```python
from build123d import *

# Parameters (mm, degrees)
BOSS_EXTRUDE1_DEPTH     = 15.21999998
SKETCH2_W               = 36.809677156
SKETCH2_H               = 26.071604974
BOSS_EXTRUDE2_DEPTH     = 3
SKETCH3_W               = 36.809677156
SKETCH3_H               = 26.071604974
BOSS_EXTRUDE3_DEPTH     = 2
SKETCH4_W               = 60.36112228
SKETCH4_H               = 157.574347664
SKETCH4_W_2             = 21
SKETCH4_H_2             = 111.767475737
CUT_EXTRUDE1_DEPTH      = 38.576
SKETCH5_W               = 10
SKETCH5_H               = 2
CUT_EXTRUDE2_DEPTH      = 38.576
SKETCH6_W               = 35.571492448
SKETCH6_H               = 20.32
CUT_EXTRUDE3_DEPTH      = 25.876
CUT_EXTRUDE3_DEPTH_BACK = 20.32
SKETCH7_W               = 25.588268566
SKETCH7_H               = 5
CUT_EXTRUDE4_DEPTH      = 25.876
SKETCH10_R              = 48.677475689
SKETCH10_R_2            = 20.5
CUT_EXTRUDE5_DEPTH      = 14.478
CUT_EXTRUDE5_DEPTH_BACK = 169.64
BOSS_EXTRUDE4_DEPTH     = 15.208
SKETCH12_W              = 30.501346117
SKETCH12_H              = 25.675497492
CUT_EXTRUDE8_DEPTH      = 8.604
CUT_EXTRUDE8_DEPTH_BACK = 0.0254
SKETCH13_W              = 21
SKETCH13_H              = 10.21999998
CUT_EXTRUDE9_DEPTH      = 8.604


with BuildPart() as part:
    # Sketch1 → Boss-Extrude1 (new body)
    with BuildSketch(Plane(origin=(0, 0, 0), x_dir=(1, 0, 0), z_dir=(0, 1, 0))):
        with BuildLine():
            Line((18.404838578, -7.300000132), (-18.404838578, -7.300000132))
            Line((-18.404838578, -7.300000132), (-18.404838578, 7.300000132))
            Line((-18.404838578, 7.300000132), (-18.404838578, 11.471604964))
            ThreePointArc((-18.404838578, 11.471604964), (0, 0), (18.404838578, 11.471604964))
            Line((18.404838578, 11.471604964), (18.404838578, 7.300000132))
            Line((18.404838578, 7.300000132), (18.404838578, -7.300000132))
        make_face()
    extrude(amount=BOSS_EXTRUDE1_DEPTH)

    # Sketch2 → Boss-Extrude2 (add)
    with BuildSketch(Plane(origin=(0, 15.21999998, 0), x_dir=(1, 0, 0), z_dir=(0, 1, 0))):
        with Locations((0, 5.735802355)):
            Rectangle(SKETCH2_W, SKETCH2_H)
    extrude(amount=-BOSS_EXTRUDE2_DEPTH)

    # Sketch3 → Boss-Extrude3 (add)
    with BuildSketch(Plane.XZ):
        with Locations((0, -5.735802355)):
            Rectangle(SKETCH3_W, SKETCH3_H)
    extrude(amount=-BOSS_EXTRUDE3_DEPTH)

    # Sketch4 → Cut-Extrude1 (cut)
    with BuildSketch(Plane.XZ):
        with Locations((0, -3.625194089)):
            Rectangle(SKETCH4_W, SKETCH4_H)
        with Locations((0, -3.62519409)):
            Rectangle(SKETCH4_W_2, SKETCH4_H_2, mode=Mode.SUBTRACT)
    extrude(amount=-CUT_EXTRUDE1_DEPTH, mode=Mode.SUBTRACT)

    # Sketch5 → Cut-Extrude2 (cut)
    with BuildSketch(Plane.XZ.offset(-12.21999998)):
        with Locations((0, -3.2352)):
            Rectangle(SKETCH5_W, SKETCH5_H)
    extrude(amount=-CUT_EXTRUDE2_DEPTH, mode=Mode.SUBTRACT)

    # Sketch6 → Cut-Extrude3 (cut, two sides)
    with BuildSketch(Plane.XZ.offset(-12.21999998)) as cut_extrude3_sk:
        with Locations((0, -18.771604842)):
            Rectangle(SKETCH6_W, SKETCH6_H)
    extrude(amount=CUT_EXTRUDE3_DEPTH, mode=Mode.SUBTRACT)
    extrude(cut_extrude3_sk.sketch, amount=-CUT_EXTRUDE3_DEPTH_BACK, mode=Mode.SUBTRACT)

    # Sketch7 → Cut-Extrude4 (cut)
    with BuildSketch(Plane(origin=(0, 15.21999998, 0), x_dir=(1, 0, 0), z_dir=(0, 1, 0))):
        with Locations((0, -7.300000132)):
            Rectangle(SKETCH7_W, SKETCH7_H)
    extrude(amount=-CUT_EXTRUDE4_DEPTH, mode=Mode.SUBTRACT)

    # Sketch10 → Cut-Extrude5 (cut, two sides)
    with BuildSketch(Plane(origin=(0, 15.21999998, 0), x_dir=(1, 0, 0), z_dir=(0, 1, 0))) as cut_extrude5_sk:
        with Locations((0, 18.199999842)):
            Circle(SKETCH10_R)
        with Locations((0, 18.199999842)):
            Circle(SKETCH10_R_2, mode=Mode.SUBTRACT)
    extrude(amount=CUT_EXTRUDE5_DEPTH, mode=Mode.SUBTRACT)
    extrude(cut_extrude5_sk.sketch, amount=-CUT_EXTRUDE5_DEPTH_BACK, mode=Mode.SUBTRACT)

    # Sketch11 → Boss-Extrude4 (add)
    with BuildSketch(Plane(origin=(0, 15.21999998, 0), x_dir=(1, 0, 0), z_dir=(0, 1, 0))):
        with BuildLine():
            Line((-10.5, 8.611604842), (10.5, 8.611604842))
            ThreePointArc((10.5, 8.611604842), (0, 11.50478798), (-10.5, 8.611604842))
        make_face()
    extrude(amount=-BOSS_EXTRUDE4_DEPTH)

    # Sketch12 → Cut-Extrude8 (cut, two sides)
    with BuildSketch(Plane.XZ) as cut_extrude8_sk:
        with Locations((1.361590216, -5.971942541)):
            Rectangle(SKETCH12_W, SKETCH12_H)
    extrude(amount=CUT_EXTRUDE8_DEPTH, mode=Mode.SUBTRACT)
    extrude(cut_extrude8_sk.sketch, amount=-CUT_EXTRUDE8_DEPTH_BACK, mode=Mode.SUBTRACT)

    # Sketch13 → Cut-Extrude9 (cut)
    with BuildSketch(Plane.XY.offset(-8.611604842)):
        with Locations((0, 7.10999999)):
            Rectangle(SKETCH13_W, SKETCH13_H)
    extrude(amount=-CUT_EXTRUDE9_DEPTH, mode=Mode.SUBTRACT)


solid = part.part
```
Check sheet for the modelled part. Datum: model origin and axes. Units: mm. A direction names the side the tool comes from. Give positions to 0.01 mm unless a question says otherwise; leave off trailing zeros. Order: outer loops, then holes, each group sorted by start corner. A loop starts at its lowest first (then second) coordinate and runs counter-clockwise, first axis right, second up. Notation, with made-up numbers: (77, -33.75) -> (103, -33.75) arc R19 ccw to (103, -10.75) -> close; hole circle Ø3 at (36, -13.75). An arc over 180 degrees is marked (long way). Use CSV: the item, a comma, the result in double quotes. Start each with the question number.
1) Mould release check, pull along Y, two halves, no side actions. Record for faces 4 (the face through (0.154, 13.741, -11.504)), 5 (the face through (0, 0.025, -5)), 6 (the face through (0, 7, 0)): released by +Y, released by -Y, zero draft, split by the parting line, or undercut.
2) Set-up check for faces 1 (the face through (0, 12.22, -6)), 2 (the face through (0.154, 1.027, -11.504)), 3 (the face through (5, 14, -3)): record each of +Z, -Z, +X, -X, +Y, -Y from which the full face is reachable in a straight line by a thin tool's end or side.
3) Sectioned sample at D-D, the plane x = 3.75. Record the boundary of the cut face in (y, z), plus the area to 3 significant figures.
4) Sectioned sample at C-C, the plane y = 13.75. Record the boundary of the cut face in (x, z).
5) Material ranges on line 1 (Y direction, x = -5.5, z = -7); line 2 (Z direction, x = -2.25, y = 12.5); line 3 (Y direction, x = 1.75, z = -4), recorded low to high. Write a range as from..to.
6) Sectioned sample at A-A, the plane z = -3.5. Record the boundary of the cut face in (x, y).
7) Sectioned sample at B-B, the plane z = -5.25. Record the boundary of the cut face in (x, y).
8) Go/stop test with flat-tipped pins: P1, Ø1.5, axis at x = -0.5, y = 14, coming from the +Z side; P2, Ø1.5, axis at x = -1.5, y = 14, coming from the -Z side; P3, Ø1.5, axis at x = -6, y = 10.5, coming from the -Z side. Record where each tip stops, or that it passes through.
Recorded:
1,face 4,"zero draft"
1,face 5,"released by -Y"
1,face 6,"undercut"
2,face 1,"-Z"
2,face 2,"-Z, +Y, -Y"
2,face 3,"+Y"
3,outline,"(0.03, -11.16) -> (2, -11.16) -> (2, -0.35) -> (12.22, -0.35) -> (12.22, -2.24) -> (15.22, -2.24) -> (15.22, 1.95) -> (0.03, 1.95) -> close; (12.22, -11.16) -> (15.22, -11.16) -> (15.22, -4.24) -> (12.22, -4.24) -> close"
3,area,"82.7 mm2"
4,outline,"(-10.5, -8.61) arc R20.5 ccw to (10.5, -8.61) -> (10.5, -0.59) arc R20.5 ccw to (-10.5, -0.59) -> close; hole (-5, -4.24) -> (5, -4.24) -> (5, -2.24) -> (-5, -2.24) -> close"
5,line 1,"0.03..2, 12.22..15.22"
5,line 2,"-11.38..-4.24, -2.24..2.18"
5,line 3,"0.03..2"
6,outline,"(-10.5, 0.03) -> (10.5, 0.03) -> (10.5, 2) -> (-10.5, 2) -> close; (-10.5, 12.22) -> (-5, 12.22) -> (-5, 15.22) -> (-10.5, 15.22) -> close; (5, 12.22) -> (10.5, 12.22) -> (10.5, 15.22) -> (5, 15.22) -> close"
7,outline,"(-10.5, 0.03) -> (10.5, 0.03) -> (10.5, 2) -> (-10.5, 2) -> close; (-10.5, 12.22) -> (10.5, 12.22) -> (10.5, 15.22) -> (-10.5, 15.22) -> close"
8,P1,"z = 2.3"
8,P2,"z = -11.49"
8,P3,"z = -1.14"
